Source: CAD feature listing. Evaluate the final solid. Frame: model axes, mm. A direction names the side the tool comes from. Give positions to 0.01 mm unless a question says otherwise; leave off trailing zeros. Loops run counter-clockwise (first coordinate to the right, second up) from the corner with the lowest first, then second, coordinate; pieces in that order, holes last. Notation, with made-up numbers: (25.25, 49.5) - (63.25, 49.5) arc R13 ccw to (63.25, 57.5) - close; hole circle Ø4 at (13.5, 17). An arc over 180 degrees is marked (long way). Put each result on its own line as item: value.
```python
from build123d import *

# Parameters (mm, degrees)
F0_W     = 700
F0_H     = 1200
F1_DEPTH = 20
F2_W     = 700
F2_H     = 320
F3_DEPTH = 110
F5_DEPTH = 680
F6_W     = 65
F6_H     = 85.7172418142
F6_H_2   = 65
F7_DEPTH = 680
F8_W     = 65
F8_H     = 65
F9_DEPTH = 570


with BuildPart() as f1:
    # F0 (on Top) → F1 (new body)
    with BuildSketch(Plane.XY):
        with Locations((252.932651341, 530.4207488894)):
            Rectangle(F0_W, F0_H)
    extrude(amount=F1_DEPTH)

    # F2 (on face) → F3 (join)
    with BuildSketch(Plane(origin=(0, 0, 0), x_dir=(1, 0, 0), z_dir=(0, 0, -1))):
        with Locations((252.932651341, -970.4207488894)):
            Rectangle(F2_W, F2_H)
    extrude(amount=F3_DEPTH)

    # F4 (on face) → F5 (cut)
    with BuildSketch(Plane(origin=(-97.067348659, 0, 0), x_dir=(0, -1, 0), z_dir=(-1, 0, 0))):
        Polygon((-830.4207488894, -55), (-830.4207488894, 0), (-1110.4207488894, 0), (-1110.4207488894, -55), (-1110.4207488894, -90), (-1005.1395893097, -90), (-830.4207488894, -90), align=None)
    extrude(amount=-F5_DEPTH, mode=Mode.SUBTRACT)

    # F6 (on face) → F7 (join)
    with BuildSketch(Plane(origin=(0, 0, 0), x_dir=(1, 0, 0), z_dir=(0, 0, -1))):
        with Locations((-64.567348659, 26.7206302035)):
            Rectangle(F6_W, F6_H)
        with Locations((570.432651341, 37.0792511106)):
            Rectangle(F6_W, F6_H_2)
    extrude(amount=F7_DEPTH)

    # F8 (on face) → F9 (join)
    with BuildSketch(Plane(origin=(0, 0, -110), x_dir=(1, 0, 0), z_dir=(0, 0, -1))):
        with Locations((-64.567348659, -1097.9207488894)):
            Rectangle(F8_W, F8_H)
        with Locations((570.432651341, -1097.9207488894)):
            Rectangle(F8_W, F8_H)
    extrude(amount=F9_DEPTH)


solid = f1.part
```
1) Mould query, pull axis Y, two halves, no side actions, for faces 4 (the flat face through (248, 1130.421, -92)), 5 (the flat face through (238, 968, 0)), 6 (the flat face through (-65, 1097, -680)). Classes: pulls with the +Y half, pulls with the -Y half, needs draft (parallel to the pull), parting line crosses it, or undercut.
Check result:
face 4: pulls with the +Y half
face 5: undercut
face 6: needs draft
2) Section query B-B, the plane z = -561.5. Output: boundary loops of the cut face in (x, y).
Check result:
outline: (-97.07, -69.58) - (-32.07, -69.58) - (-32.07, 16.14) - (-97.07, 16.14) - close; (-97.07, 1065.42) - (-32.07, 1065.42) - (-32.07, 1130.42) - (-97.07, 1130.42) - close; (537.93, -69.58) - (602.93, -69.58) - (602.93, -4.58) - (537.93, -4.58) - close; (537.93, 1065.42) - (602.93, 1065.42) - (602.93, 1130.42) - (537.93, 1130.42) - close
3) Section query C-C, the plane y = 844. Output: boundary loops of the cut face in (x, z).
Check result:
outline: (-97.07, -110) - (602.93, -110) - (602.93, 20) - (-97.07, 20) - (-97.07, 0) - (582.93, 0) - (582.93, -90) - (-97.07, -90) - close
4) Section query A-A, the plane x = 320. Output: boundary loops of the cut face in (y, z).
Check result:
outline: (-69.58, 0) - (810.42, 0) - (810.42, -110) - (1130.42, -110) - (1130.42, 20) - (-69.58, 20) - close; hole (830.42, -90) - (1110.42, -90) - (1110.42, 0) - (830.42, 0) - close
5) Pin query (flat end, axial travel): P1, Ø1, axis at x = 186.5, y = 271.5, coming from the -Z side. Return the tip coordinate at first contact, or that it passes through.
Check result:
P1: z = 0
6) Section query D-D, the plane y = 71.5. Output: boundary loops of the cut face in (x, z), plus the area to 3 significant figures.
Check result:
outline: (-97.07, 0) - (602.93, 0) - (602.93, 20) - (-97.07, 20) - close
area: 14,000 mm²
7) Material intervals for line 1 along Z through (x, y) = (139.5, 989); line 2 along X through (y, z) = (1067, -125); line 3 along Y through (x, z) = (-24, -85.5), sorted ascending. Write a range as [from, to].
Check result:
line 1: [-110, -90], [0, 20]
line 2: [-97.07, -32.07], [537.93, 602.93]
line 3: [810.42, 830.42], [1110.42, 1130.42]
8) Access query for faces 1 (the flat face through (582.933, 972, -44)), 2 (the flat face through (-65, 1065.421, -391)), 3 (the flat face through (570, -4.579, -335)). Directions: +Z, -Z, +X, -X, +Y, -Y. A direction counts if a zero-diameter tool reaches every point of the face in a straight line with its end or side. Return the directions, or none.
Check result:
face 1: -X
face 2: -Z, +X, -X
face 3: -Z, +X
